Could you check a few things on this model? Use its own coordinates, in mm. Face numbers are marked on the shaded views. Coordinates: 2 decimals unless noted, no trailing zeros. Order: outer loops, then holes, each group sorted by start corner. A loop starts at its lowest first (then second) coordinate and runs counter-clockwise, first axis right, second up. Notation, with made-up numbers: (53, -38.75) - (88, -38.75) arc R25 cw to (88, -26.75) - close; hole circle Ø2 at (-13, 87.5). An arc over 180 degrees is marked (long way). Answer as CSV lines item,"result". Start each with the question number.
1. I need wall thicknesses on probe 1 along Y at (x, z) = (0, 9.25); probe 2 along X at (y, z) = (50, 9.5); probe 3 along X at (y, z) = (25, 8.25). Which ranges of each line are inside material? Lowest first, please.
2. For pin 1 (8 mm diameter, centred on x = -2, z = 11.5, fed in from +Y); pin 2 (1.5 mm diameter, centred on y = 25, z = 5.5, fed in from +X); pin 3 (1 mm diameter, centred on x = 38, z = 11.5, fed in from +Y), each with a flat end and sliding along its axis, tell me the tip position at first contact or that it passes through.
3. I want a section at A-A, the plane x = 0. List the corners of the cut face in (y, z) for me, and give its area (3 significant figures).
4. I want a section at C-C, the plane z = 5.75. List the corners of the cut face in (x, y) for me, and give its area (3 significant figures).
5. I want a section at B-B, the plane y = 0. List the corners of the cut face in (x, z) for me, and give its area (3 significant figures).
6. Thinking about a two-plate mould opening in X: for the marked faces 1, 2, 3 and 4, which applies, released by +X, released by -X, zero draft, split by the parting line, or undercut?
from build123d import *

# Parameters (mm, degrees)
F0_R     = 57.65
F1_DEPTH = 15


with BuildPart() as f1:
    # F0 (on Top) → F1 (new body)
    with BuildSketch(Plane.XY):
        with BuildLine():
            Line((71.727416, 16.873064), (44.30024, 44.30024))
            ThreePointArc((44.30024, 44.30024), (0, 62.65), (-44.30024, 44.30024))
            Line((-44.30024, 44.30024), (-71.727416, 16.873064))
            ThreePointArc((-71.727416, 16.873064), (-75.876353, 10.82022), (-77.562828, 3.678344))
            ThreePointArc((-77.562828, 3.678344), (-77.65, 0), (-77.562828, -3.678344))
            ThreePointArc((-77.562828, -3.678344), (-75.876353, -10.82022), (-71.727416, -16.873064))
            Line((-71.727416, -16.873064), (-44.30024, -44.30024))
            ThreePointArc((-44.30024, -44.30024), (0, -62.65), (44.30024, -44.30024))
            Line((44.30024, -44.30024), (71.727416, -16.873064))
            ThreePointArc((71.727416, -16.873064), (75.876353, -10.82022), (77.562828, -3.678344))
            ThreePointArc((77.562828, -3.678344), (77.65, 0), (77.562828, 3.678344))
            ThreePointArc((77.562828, 3.678344), (75.876353, 10.82022), (71.727416, 16.873064))
        make_face()
        Circle(F0_R, mode=Mode.SUBTRACT)
    extrude(amount=F1_DEPTH)


solid = f1.part
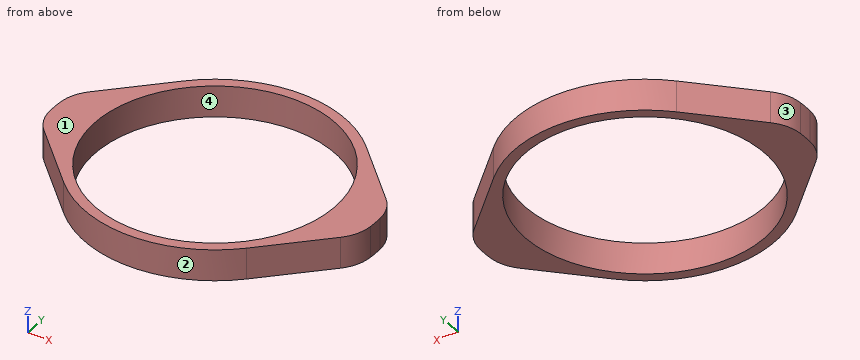
Solved:
1,probe 1,"y = -62.65 to -57.65, 57.65 to 62.65"
1,probe 2,"x = -37.75 to -28.7, 28.7 to 37.75"
1,probe 3,"x = -63.6 to -51.95, 51.95 to 63.6"
2,pin 1,"stops at y = 62.65"
2,pin 2,"stops at x = 64.35"
2,pin 3,"stops at y = 50.19"
3,outline,"(-62.65, 0) - (-57.65, 0) - (-57.65, 15) - (-62.65, 15) - close; (57.65, 0) - (62.65, 0) - (62.65, 15) - (57.65, 15) - close"
3,area,"150 mm2"
4,outline,"(-77.56, -3.68) arc R20 ccw to (-71.73, -16.87) - (-44.3, -44.3) arc R62.65 ccw to (44.3, -44.3) - (71.73, -16.87) arc R20 ccw to (77.56, -3.68) arc R77.65 ccw to (77.56, 3.68) arc R20 ccw to (71.73, 16.87) - (44.3, 44.3) arc R62.65 ccw to (-44.3, 44.3) - (-71.73, 16.87) arc R20 ccw to (-77.56, 3.68) arc R77.65 ccw to start; hole circle Ø115.3 at (0, 0)"
4,area,"3,300 mm2"
5,outline,"(-77.65, 0) - (-57.65, 0) - (-57.65, 15) - (-77.65, 15) - close; (57.65, 0) - (77.65, 0) - (77.65, 15) - (57.65, 15) - close"
5,area,"600 mm2"
6,face 1,"zero draft"
6,face 2,"split by the parting line"
6,face 3,"released by -X"
6,face 4,"undercut"
